Read the model definition and answer for the solid it produces. Units are mm, in the model's axes. A direction names the side the tool comes from. Coordinates: 2 decimals unless noted, no trailing zeros. Order: outer loops, then holes, each group sorted by start corner. A loop starts at its lowest first (then second) coordinate and runs counter-clockwise, first axis right, second up.
from build123d import *

# Parameters (mm, degrees)
EXTRUDE_1_DEPTH     = 32
CHAMFER_1_SIZE      = 2
CUT_EXTRUDE_1_DEPTH = 22
SKETCH_3_W          = 8
SKETCH_3_H          = 28
CUT_EXTRUDE_2_DEPTH = 7.2
CHAMFER_2_SIZE      = 2.5


with BuildPart() as part:
    # Эскиз1 → Бобышка-Вытянуть1 (new body)
    with BuildSketch(Plane.XY):
        Polygon((0, 10), (0, 0), (10, 0), (10, -5), (-5, -5), (-5, 10), align=None)
    extrude(amount=EXTRUDE_1_DEPTH)

    # Фаска1
    chamfer_1_edges = [part.edges().sort_by_distance(p)[0] for p in [
        (-5, -5, 16),
    ]]
    chamfer(chamfer_1_edges, length=CHAMFER_1_SIZE)

    # Эскиз2 → Вырез-Вытянуть1 (cut)
    with BuildSketch(Plane.XY.offset(32)):
        Polygon((-2, -2), (-2, 10), (-5, 10), (-5, -3), (-3, -5), (10, -5), (10, -2), align=None)
    extrude(amount=-CUT_EXTRUDE_1_DEPTH, mode=Mode.SUBTRACT)

    # Эскиз3 → Вырез-Вытянуть2 (cut)
    with BuildSketch(Plane(origin=(-4, -4, 0), x_dir=(0, 0, 1), z_dir=(-0.707106781, -0.707106781, 0))):
        with Locations((19, 0)):
            Rectangle(SKETCH_3_W, SKETCH_3_H)
    extrude(amount=-CUT_EXTRUDE_2_DEPTH, mode=Mode.SUBTRACT)

    # Фаска2
    chamfer_2_edges = [part.edges().sort_by_distance(p)[0] for p in [
        (-2, -2, 12.5),
        (-2, -2, 27.5),
    ]]
    chamfer(chamfer_2_edges, length=CHAMFER_2_SIZE)

    # Эскиз4 → Отверстие обработанное метчиком #4-401 (revolve, cut)
    with BuildSketch(Plane(origin=(-2, -2, 0), x_dir=(0, 1, 0), z_dir=(1, 0, 0))):
        Polygon((0, 0), (0, 10), (1.651, 10), (1.4224, 9.839932557), (1.4224, 0.160067443), (1.651, 0), align=None)
    revolve(axis=Axis((-2, -2, -6.35), (0, 0, 1)), mode=Mode.SUBTRACT)


solid = part.part
Q1. The part is cut by section C-C, the plane z = 7. Determine the outline of the cut face in (x, y), then the cut area to 3 significant figures.
Q2. Which of the six approach directions +Z, -Z, +X, -X, +Y, -Y give full straight-line access (tool end or side, diameter ignored) to faces 1 (the flat face through (5, -2, 21)), 2 (the flat face through (-1.014, 3.196, 18.944)), 3 (the flat face through (0, -2, 10))?
Q3. The part is cut by section B-B, the plane y = 1. Determine the outline of the cut face in (x, z), then the cut area to 3 significant figures.
Q4. Straight lines are drawn through the part: L1, parallel to Y at x = -2, z = 6; L2, parallel to Y at x = 8.25, z = 11. For each, find the intervals that lie inside material, in ascending order.
Q5. The part is cut by section A-A, the plane z = 17. Determine the outline of the cut face in (x, y), then the cut area to 3 significant figures.
Q6. Determine the mould class of faces 4 (the flat face through (4, -5, 5)), 5 (the cylindrical face through (-2.06, -3.42, 4.93)), 6 (the flat face through (10, -1, 12)), 7 (the flat face through (3.17, -0.99, 18.94)) for opening direction X: +X half, -X half, draft (parallel to the pull), parting line (faces both ways), or undercut.
Q7. Each of these flat-tipped pins is pushed along its axis until it touches: P1, Ø2.5, axis at x = -2, y = -2, coming from the +Z side; P2, Ø1, axis at x = 8, z = 17.5, coming from the +Y side; P3, Ø2, axis at y = 1.5, z = 17, coming from the -X side; P4, Ø8, axis at x = 5.5, z = 20, coming from the -Y side. Where does it stop, or does it pass through?
Computed values:
1. outline: (-5, -3) - (-3, -5) - (10, -5) - (10, 0) - (0, 0) - (0, 10) - (-5, 10) - close; hole circle Ø2.84 at (-2, -2)
1. area: 117 mm2
2. face 1: +Z, +X, -X, -Y
2. face 2: -X, -Y
2. face 3: +Z, -X, -Y
3. outline: (-5, 0) - (0, 0) - (0, 15) - (-2, 15) - (-2, 10) - (-5, 10) - close; (-2, 23) - (0, 23) - (0, 32) - (-2, 32) - close
3. area: 78.0 mm2
4. L1: y = -5 to -3.42, -0.58 to 10
4. L2: y = -2 to 0
5. outline: (-2, 4.18) - (0, 2.18) - (0, 10) - (-2, 10) - close; (2.18, 0) - (4.18, -2) - (10, -2) - (10, 0) - close
5. area: 27.3 mm2
6. face 4: draft
6. face 5: undercut
6. face 6: +X half
6. face 7: -X half
7. P1: passes through
7. P2: stops at y = 0
7. P3: stops at x = -0.32
7. P4: stops at y = -2
